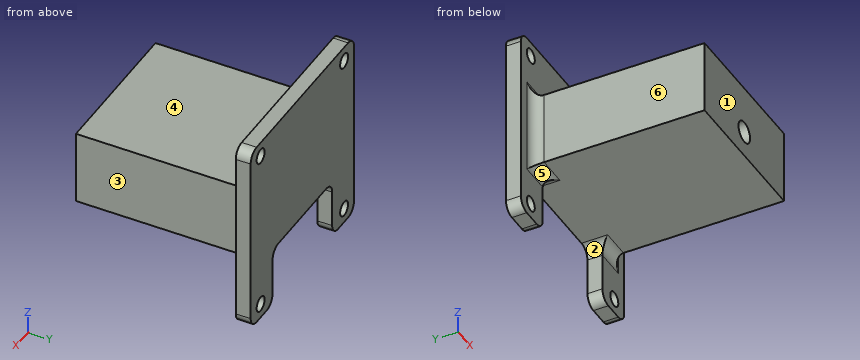
```python
from build123d import *

# Parameters (mm, degrees)
SKETCH_1_W          = 20
SKETCH_1_H          = 10
SKETCH_1_R          = 1.45
EXTRUDE_1_DEPTH     = 23
SKETCH_2_R          = 1
EXTRUDE_2_DEPTH     = 2
SKETCH_3_W          = 15
SKETCH_3_H          = 16
CUT_EXTRUDE_1_DEPTH = 15
FILLET_3_R          = 1.5


with BuildPart() as part:
    # 草图1 → 凸台-拉伸1 (new body)
    with BuildSketch(Plane(origin=(0, 0, 0), x_dir=(1, 0, 0), z_dir=(0, 1, 0))):
        Rectangle(SKETCH_1_W, SKETCH_1_H)
        with Locations(Location((0, 1.5, 0), (0, 0, 270))):
            Circle(SKETCH_1_R, mode=Mode.SUBTRACT)
    extrude(amount=EXTRUDE_1_DEPTH)

    # 草图2 → 凸台-拉伸2 (add)
    with BuildSketch(Plane(origin=(0, 23, 0), x_dir=(1, 0, 0), z_dir=(0, 1, 0))):
        Polygon((13, -13), (0, -13), (-13, -13), (-13, 13), (13, 13), align=None)
        with Locations(Location((-10.5, 11, 0), (0, 0, 270))):
            Circle(SKETCH_2_R, mode=Mode.SUBTRACT)
        with Locations(Location((10.5, 11, 0), (0, 0, 90))):
            Circle(SKETCH_2_R, mode=Mode.SUBTRACT)
        with Locations(Location((10.5, -11, 0), (0, 0, 270))):
            Circle(SKETCH_2_R, mode=Mode.SUBTRACT)
        with Locations(Location((-10.5, -11, 0), (0, 0, 90))):
            Circle(SKETCH_2_R, mode=Mode.SUBTRACT)
    extrude(amount=EXTRUDE_2_DEPTH)

    # 草图3 → 切除-拉伸1 (cut)
    with BuildSketch(Plane(origin=(0, 25, 0), x_dir=(1, 0, 0), z_dir=(0, 1, 0))):
        with Locations((0, 13)):
            Rectangle(SKETCH_3_W, SKETCH_3_H)
    extrude(amount=-CUT_EXTRUDE_1_DEPTH, mode=Mode.SUBTRACT)

    # 圆角3
    fillet_3_edges = [part.edges().sort_by_distance(p)[0] for p in [
        (10, 23, 0),
        (8.75, 23, -5),
        (-13, 24, -13),
        (-13, 24, 13),
        (13, 24, 13),
        (13, 24, -13),
        (7.5, 24, -13),
        (-7.5, 24, -13),
        (-8.75, 23, -5),
        (7.5, 24, -5),
        (-7.5, 24, -5),
        (-10, 23, 0),
        (0, 23, 5),
    ]]
    fillet(fillet_3_edges, radius=FILLET_3_R - 0.0001)  # a hair under: the kernel refuses the full size


solid = part.part
```
Input: part model. Units: mm. Frame: model coordinates. Face numbers are marked on the shaded views. A direction names the side the tool comes from. Give positions to 0.01 mm unless a question says otherwise; leave off trailing zeros. Loops run counter-clockwise (first coordinate to the right, second up) from the corner with the lowest first, then second, coordinate; pieces in that order, holes last.
1) Section query A-A on z = -11. Return the cut outline in (x, y).
A:
outline: (-13, 23) - (-11.5, 23) - (-11.5, 25) - (-13, 25) - close; (-9.5, 23) - (-7.5, 23) - (-7.5, 25) - (-9.5, 25) - close; (7.5, 23) - (9.5, 23) - (9.5, 25) - (7.5, 25) - close; (11.5, 23) - (13, 23) - (13, 25) - (11.5, 25) - close
2) Mould query, pull axis X, two halves, no side actions, for the marked faces 1, 2 and 3. Classes: released by +X, released by -X, zero draft, split by the parting line, or undercut.
A:
face 1: zero draft
face 2: undercut
face 3: released by +X
3) Section query B-B on z = -7.5. Return the cut outline in (x, y), and give its area (3 significant figures).
A:
outline: (-13, 23) - (-7.5, 23) - (-7.5, 25) - (-13, 25) - close; (7.5, 23) - (13, 23) - (13, 25) - (7.5, 25) - close
area: 22.0 mm2
4) Line query: L1, parallel to X at y = 23.65, z = -11; L2, parallel to X at y = 23.6, z = 11; L3, parallel to Y at x = -5, z = 6.5. Output: solid intervals per line, ascending.
A:
L1: x = -13 to -11.5, -9.5 to -7.5, 7.5 to 9.5, 11.5 to 13
L2: x = -13 to -11.5, -9.5 to 9.5, 11.5 to 13
L3: y = 23 to 25
5) Section query D-D on x = -2. Return the cut outline in (y, z), and give its area (3 significant figures).
A:
outline: (0, -5) - (25, -5) - (25, 13) - (23, 13) - (23, 6.5) arc R1.5 cw to (21.5, 5) - (0, 5) - close
area: 266 mm2
6) Reachability of the marked faces 4, 5 and 6 from +Z, -Z, +X, -X, +Y, -Y: full face, straight path, thin tool, end or side. Return the list, or none.
A:
face 4: +Z, +X, -X, -Y
face 5: -Z, +X, -X, -Y
face 6: +Z, -Z, -X, -Y
7) Contact query for flat-ended pins moving along their axis: pin 1 (10 mm diameter, centred on y = 5, z = -3.5, fed in from -X); pin 2 (3 mm diameter, centred on x = -10.5, z = 11, fed in from +Y); pin 3 (12 mm diameter, centred on x = -8.5, y = 9.5, fed in from -Z); pin 4 (12 mm diameter, centred on y = 16, z = -4.5, fed in from -X). Output: stop coordinate, or through.
A:
pin 1: stops at x = -10
pin 2: stops at y = 25
pin 3: stops at z = -5
pin 4: stops at x = -10.09
8) Section query C-C on y = 8.5. Return the cut outline in (x, z).
A:
outline: (-10, -5) - (10, -5) - (10, 5) - (-10, 5) - close; hole circle Ø2.9 at (0, -1.5)
